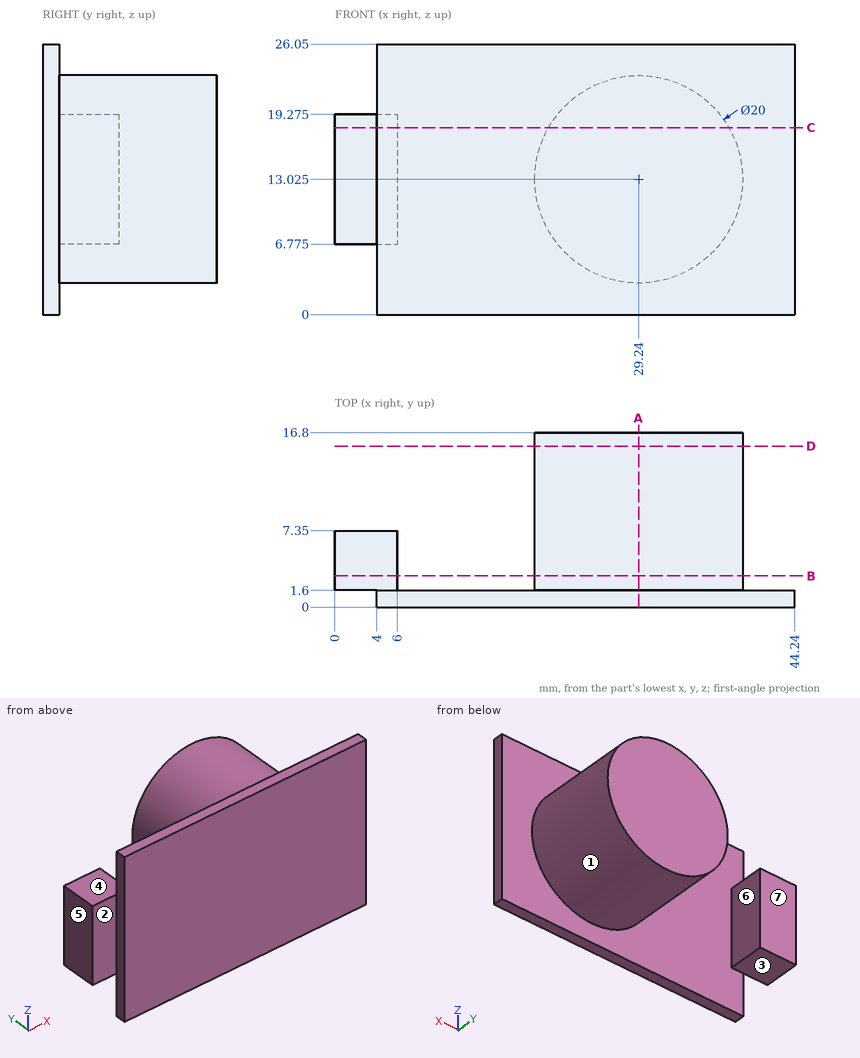
For this review, use the dimensioned drawing (mm, ordinates from the lowest corner) and the shaded views. A direction names the side the tool comes from. Round coordinates to 2 decimals unless told otherwise and drop trailing zeros. Write each loop counter-clockwise with the first axis right and the second up, starting at its lowest first coordinate (ties: lowest second). Pieces come first, ordered by that corner, then holes. Notation, with made-up numbers: (21, 42) -> (74, 42) arc R21 cw to (74, 54) -> close; hole circle Ø2 at (24, -25). An arc over 180 degrees is marked (long way). Answer in a Markdown table with one row per item.
Q1. For the marked faces 1, 2, 3 and 4, list the 3-axis set-ups (+Z, -Z, +X, -X, +Y, -Y) from which the entire face can be reached by the end or side of a thin tool; tool diameter is ignored.
The answers:
| item | result |
|---|---|
| face 1 | +Y |
| face 2 | +Z, -Z, -X, -Y |
| face 3 | -Z, -X, +Y |
| face 4 | +Z, -X, +Y |
Q2. To check wall thickness, follow L1, parallel to Y at x = 39.5, z = 14.25; L2, parallel to Z at x = 4.5, y = 4.25 (3 decimals); L3, parallel to X at y = 5, z = 13.75. State the ranges of each line that lie inside material, in increasing order. Write a range as [from, to].
The answers:
| item | result |
|---|---|
| L1 | [0, 1.6] |
| L2 | [6.775, 19.275] |
| L3 | [0, 6], [19.27, 39.21] |
Q3. Take a section at A-A, the plane x = 29.24. State the section outline as (y, z) points (3 decimals), then the cut area to 3 significant figures.
The answers:
| item | result |
|---|---|
| outline | (0, 0) -> (1.6, 0) -> (1.6, 3.025) -> (16.8, 3.025) -> (16.8, 23.025) -> (1.6, 23.025) -> (1.6, 26.05) -> (0, 26.05) -> close |
| area | 346 mm² |
Q4. Take a section at D-D, the plane y = 15.5. State the section outline as (x, z) points (3 decimals), then the cut area to 3 significant figures.
The answers:
| item | result |
|---|---|
| outline | circle Ø20 at (29.24, 13.025) |
| area | 314 mm² |
Q5. Clearance check with flat-ended pins moving along their axes: pin 1 Ø6 at (x, y) = (28, 13.5) entering from +Z (3 decimals); pin 2 Ø2 at (y, z) = (8, 21) entering from -X; pin 3 Ø8 at (x, y) = (19.5, 13.5) entering from +Z; pin 4 Ø10 at (x, z) = (30, 16) entering from -Y. State where each tip first meets the part, or that it passes through.
The answers:
| item | result |
|---|---|
| pin 1 | z = 23.025 |
| pin 2 | x = 22.07 |
| pin 3 | z = 21.21 |
| pin 4 | y = 0 |
Q6. Draft analysis for pull direction X (two halves, no side actions). For the marked faces 5, 6 and 7, state which applies: +X half, -X half, draft (parallel to the pull), parting line (faces both ways), or undercut.
The answers:
| item | result |
|---|---|
| face 5 | -X half |
| face 6 | undercut |
| face 7 | draft |
Q7. Take a section at B-B, the plane y = 3. State the section outline as (x, z) points (3 decimals), then the cut area to 3 significant figures.
The answers:
| item | result |
|---|---|
| outline | (0, 6.775) -> (6, 6.775) -> (6, 19.275) -> (0, 19.275) -> close; circle Ø20 at (29.24, 13.025) |
| area | 389 mm² |
Q8. Take a section at C-C, the plane z = 18. State the section outline as (x, y) points.
The answers:
| item | result |
|---|---|
| outline | (0, 1.6) -> (4, 1.6) -> (4, 0) -> (44.24, 0) -> (44.24, 1.6) -> (37.91, 1.6) -> (37.91, 16.8) -> (20.57, 16.8) -> (20.57, 1.6) -> (6, 1.6) -> (6, 7.35) -> (0, 7.35) -> close |
